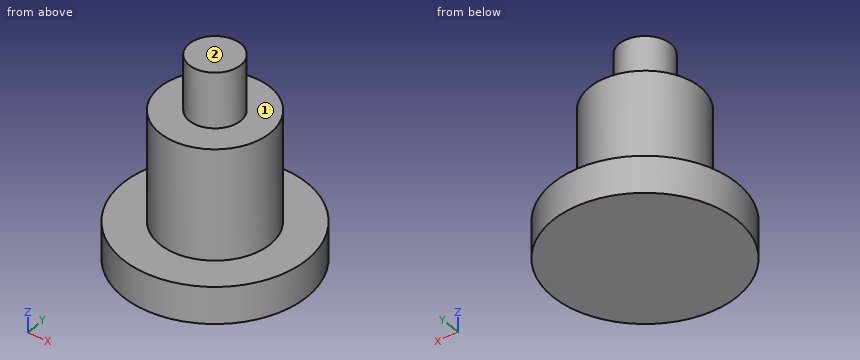
Autodesk Fusion 360 part; units mm, degrees
sketch "Sketch1" plane through (0, 0, 0) normal (0, 0, 1) x (1, 0, 0)
  circle A0 centre (0, 0) radius 5
  circle A1 centre (0, 0) radius 3
  circle A2 centre (0, 0) radius 1.4
  dimension "d1" = 10
  dimension "d2" = 6
  dimension "d3" = 2.8
extrude "Extrude1" add sketch "Sketch1" along normal blind 2 contours A0 | A1 | A2
extrude "Extrude2" add sketch "Sketch1" along normal blind 8 contours A1 | A2
extrude "Extrude3" add sketch "Sketch1" along normal blind 11 contours A2
Can you work these out from the model? Positions are in its coordinate system, mm. Face numbers are marked on the shaded views. A direction names the side the tool comes from. Round coordinates to 2 decimals unless told otherwise and drop trailing zeros. Order: outer loops, then holes, each group sorted by start corner. A loop starts at its lowest first (then second) coordinate and runs counter-clockwise, first axis right, second up.
(1) If we section it at C-C (z = 5.5): Please give me the cut outline in (x, y), plus the area to 3 significant figures.
Results are:
outline: circle Ø6 at (0, 0)
area: 28.3 mm2
(2) On a 3-axis mill with a long thin cutter (end or side, diameter ignored), from which of +Z, -Z, +X, -X, +Y, -Y can I reach the whole of each face in a straight line? I mean the marked faces 1 and 2. Say none if no direction works.
Results are:
face 1: +Z
face 2: +Z, +X, -X, +Y, -Y
(3) If we section it at D-D (x = 1.75): Please give me the cut outline in (y, z), plus the area to 3 significant figures.
Results are:
outline: (-4.68, 0) - (4.68, 0) - (4.68, 2) - (2.44, 2) - (2.44, 8) - (-2.44, 8) - (-2.44, 2) - (-4.68, 2) - close
area: 48.0 mm2
(4) If we section it at A-A (y = 0): Please give me the cut outline in (x, z), plus the area to 3 significant figures.
Results are:
outline: (-5, 0) - (5, 0) - (5, 2) - (3, 2) - (3, 8) - (1.4, 8) - (1.4, 11) - (-1.4, 11) - (-1.4, 8) - (-3, 8) - (-3, 2) - (-5, 2) - close
area: 64.4 mm2
(5) I'm going to push flat-ended pins straight in: pin 1 (4 mm diameter, centred on y = -1, z = 8.5, fed in from -X); pin 2 (3 mm diameter, centred on x = 1, z = 6, fed in from -Y); pin 3 (3 mm diameter, centred on x = -2, y = -3, fed in from +Z). Where does each tip first touch, or does it pass through?
Results are:
pin 1: stops at x = -3
pin 2: stops at y = -3
pin 3: stops at z = 8
(6) If I drill on L1, parallel to Z at x = -4, y = 2.25; L2, parallel to X at y = 0, z = 6.75; L3, parallel to Y at x = 0, z = 9, over which ranges is the centre line in solid material (lowest first)?
Results are:
L1: z = 0 to 2
L2: x = -3 to 3
L3: y = -1.4 to 1.4
